Geometry check sheet. Reference: the model listing, model coordinates, mm. A direction names the side the tool comes from. Round coordinates to 2 decimals unless told otherwise and drop trailing zeros. Loops run counter-clockwise (first coordinate to the right, second up) from the corner with the lowest first, then second, coordinate; pieces in that order, holes last. Notation, with made-up numbers: (-33, -22.5) - (13, -22.5) arc R33 ccw to (13, 14.5) - close; hole circle Ø4 at (81.5, -21). An arc over 180 degrees is marked (long way). Answer in a Markdown table with one row per item. Add a question column.
Autodesk Inventor part; units mm, degrees
ref_plane "Work Plane2" through (3.35, 0, 0) normal (0, 0, -1) x (1, 0, 0)
ref_plane "YZ Plane" through (0, 0, 0) normal (1, 0, 0) x (0, 1, 0)
ref_plane "XZ Plane" through (0, 0, 0) normal (0, 1, 0) x (-1, 0, 0)
sketch "Szkic1" plane through (0, 0, 0) normal (0, 0, 1) x (1, 0, 0)
  line L0 (1.76, 0) -> (8, 0)
  line L1 (8, 0) -> (8, 1.5)
  line L2 (8, 1.5) -> (2.65, 1.5)
  line L3 (2.65, 1.5) -> (2.3433, 1.3466)
  line L4 (2.3433, 1.3466) -> (1.65, 1.3466)
  line L5 (0, 2.65) -> (0, 1.525)
  line L6 (0, 1.525) -> (1.2915, 0.8811)
  line L7 (1.2915, 0.8811) -> (1.76, 0)
  line L8 (-1.6, 0) -> (9.6, 0)
  line L9 (0, -0.53) -> (0, 3.18)
  line L10 (0, 2.65) -> (0.3466, 2.65)
  line L11 (0.3466, 2.65) -> (1.65, 1.3466)
  line L12 (2.65, 1.5) -> (1.4966, 1.5) construction
  dimension "d1" = 5.35
  dimension "d2" = 3
  dimension "d3" = 2.6933
  dimension "d4" = 3.05
  dimension "d5" = 26.5
  dimension "d6" = 62
  dimension "d7" = 1.76
  dimension "d8" = 0.3067
  dimension "d12" = 5.3
  dimension "d13" = 45
  dimension "d15" = 8
  dimension "d24" = 1.65
revolve "Bryła" add sketch "Szkic1" angle 360 about axis through (1.76, 0, 0) along (1, 0, 0) contours L7 L6 L5 L10 L11 L4 L3 L2 L1 L0
sketch "Szkic2" plane through (0, 0, 0) normal (-1, 0, 0) x (0, 0, 1)
  line L0 (0, 1.525) -> (0, 0) construction
  line L1 (0, 0) -> (1.525, 0) construction
  arc A0 (0.4575, 0) -> (0, 0.4575) centre (0, 0) ccw construction
  arc A1 (0.5338, 0) -> (0, 0.5337) centre (0, 0) ccw construction
  arc A2 (1.4843, 0.35) -> (0.35, 1.4843) centre (0, 0) ccw
  line L2 (0, 0) -> (1.0783, 1.0783) construction
  line L3 (0.35, 1.4843) -> (0.2734, 0.4584)
  line L4 (1.4843, 0.35) -> (0.4584, 0.2734)
  arc A3 (0.35, 1.4843) -> (0, 1.525) centre (0, 0) ccw
  arc A4 (1.525, 0) -> (1.4843, 0.35) centre (0, 0) ccw
  line L5 (0, -3.71) -> (0, 3.71)
  line L6 (-3.71, 0) -> (3.71, 0)
  arc A5 (0.35, -1.4843) -> (1.4843, -0.35) centre (0, 0) ccw
  line L7 (0.35, -1.4843) -> (0.2734, -0.4584)
  line L8 (1.4843, -0.35) -> (0.4584, -0.2734)
  arc A6 (0, -1.525) -> (0.35, -1.4843) centre (0, 0) ccw
  arc A7 (1.4843, -0.35) -> (1.525, 0) centre (0, 0) ccw
  arc A8 (-0.35, 1.4843) -> (-1.4843, 0.35) centre (0, 0) ccw
  line L9 (-0.35, 1.4843) -> (-0.2734, 0.4584)
  line L10 (-1.4843, 0.35) -> (-0.4584, 0.2734)
  arc A9 (0, 1.525) -> (-0.35, 1.4843) centre (0, 0) ccw
  arc A10 (-1.4843, 0.35) -> (-1.525, 0) centre (0, 0) ccw
  arc A11 (-0.35, -1.4843) -> (0, -1.525) centre (0, 0) ccw
  arc A12 (-1.4843, -0.35) -> (-0.35, -1.4843) centre (0, 0) ccw
  arc A13 (-1.525, 0) -> (-1.4843, -0.35) centre (0, 0) ccw
  line L11 (-1.4843, -0.35) -> (-0.4584, -0.2734)
  line L12 (-0.35, -1.4843) -> (-0.2734, -0.4584)
  arc A14 (0.2734, 0.4584) -> (0.4584, 0.2734) centre (0.4455, 0.4455) ccw
  arc A15 (0.4584, -0.2734) -> (0.2734, -0.4584) centre (0.4455, -0.4455) ccw
  arc A16 (-0.4584, 0.2734) -> (-0.2734, 0.4584) centre (-0.4455, 0.4455) ccw
  arc A17 (-0.2734, -0.4584) -> (-0.4584, -0.2734) centre (-0.4455, -0.4455) ccw
  point P0 (1.0783, -1.0783)
  point P1 (-1.0783, 1.0783)
  point P2 (-1.0783, -1.0783)
  dimension "d17" = 0.915
  dimension "d18" = 1.0675
  dimension "d19" = 3.05
  dimension "d20" = 45
  dimension "d21" = 0.35
extrude "Szczelina" add sketch "Szkic2" against normal up to next draft 5 contours L4 A14 L3 A2 | A5 L7 A15 L8 | L9 A16 L10 A8 | A12 L11 A17 L12
fillet "Zaokrąglenie1" radius 0.14 4 edges at (0, 1.525, 0) (0, 0, -1.525) (0, -1.525, 0) (0, 0, 1.525)
thread "Gwint"
chamfer "Faza1" distance 0.3067 distance2 0.1534 1 edges at (8, -1.5, 0) measured on face at (8, 0.3888, 0.4512)
ref_plane "Work Plane2" through (3.35, 0, 0) normal (0, 0, -1) x (1, 0, 0)
equation "\"d1\" = GEL"
equation "\"d2\" = GD"
equation "\"d3\" = BDM"
equation "\"d4\" = SDM"
equation "\"d7\" = INTI"
equation "\"d8\" = GAL"
equation "\"d12\" = KOD"
equation "\"d13\" = 0.5 * SEWI"
equation "\"d15\" = NLG"
equation "\"d24\" = KOH"
equation "\"d17\" = 0.3 * SDM"
equation "\"d18\" = 0.35 * SDM"
equation "\"d19\" = SDM"
equation "\"d21\" = 0.5 * SBR"
equation "\"d23\" = 0.2 * SBR"
equation "\"d10\" = GEL"
equation "\"d25\" = -0.5 * SPD + 0.5 * GD"
equation "\"d26\" = 0.5 * GAL"
equation "\"NLG\" = 8"
equation "\"GEL\" = 5.35"
equation "\"GAL\" = 0.61345 * PTC"
equation "\"SPD\" = NND - 1.2269 * PTC"
equation "\"KOD\" = 5.3"
equation "\"KOH\" = 1.65"
equation "\"SBR\" = 0.7"
equation "\"INTI\" = 1.76"
equation "\"SDM\" = 3.05"
equation "\"GD\" = NND"
equation "\"BDM\" = NND - GAL"
equation "\"SEWI\" = 90deg"
equation "\"d9\" = SDM"
equation "\"GUL\" = 0.61345 * PTC"
equation "\"TOA\" = 30deg"
equation "\"EPV\" = 3.15"
equation "\"THREADDIA\" = 3"
equation "\"RR\" = 0.3"
equation "\"PTC\" = 0.5"
equation "\"NND\" = 3"
equation "\"GD1\" = THREADDIA - 1.2269 * PTC"
properties part number "AS 1427 - M3 x 8" material "Stal, miękka"
Q1. Set-up check for faces 4 (the cylindrical face through (5.21, -1.5, -0.07)), 5 (the flat face through (0.573, -0.247, -0.779)), 6 (the flat face through (8, 0, 0)): record each of +Z, -Z, +X, -X, +Y, -Y from which the full face is reachable in a straight line by a thin tool's end or side.
Q2. Scan lines: line 1 (X direction, y = -1.6, z = -0.4); line 2 (Y direction, x = 3.5, z = 0.2); line 3 (Z direction, x = 1.5, y = 0.25). Record each from-to range of solid material in increasing order. Write a range as from..to.
Q3. Cross-section at A-A, the plane x = 1. Enter the section's corners in (y, z), plus the area to 3 significant figures.
Q4. Release check for a two-part mould opening along Y. For faces 1 (the flat face through (0.573, 0.779, 0.247)), 2 (the cylindrical face through (1.992, -1.345, -0.059)), 3 (the flat face through (0, 1, -1)) record: +Y half, -Y half, draft (parallel to the pull), parting line (faces both ways), or undercut.
Q5. Cross-section at B-B, the plane x = 3.75. Enter the section's corners in (y, z).
Q6. Depth check by flat-ended pin: P1, Ø1.5, axis at x = 4.5, z = -2, coming from the +Y side; P2, Ø1.5, axis at y = 1, z = -1.5, coming from the -X side; P3, Ø1, axis at x = 5, z = -0.5, coming from the -Y side. Enter the tip coordinate at first touch or a pass-through.
Check sheet entries:
| question | item | result |
|---|---|---|
| 1 | face 4 | +X |
| 1 | face 5 | -X |
| 1 | face 6 | +Z, -Z, +X, +Y, -Y |
| 2 | line 1 | 0..1.35 |
| 2 | line 2 | -1.49..1.49 |
| 2 | line 3 | -1.48..-0.21, 0.21..1.48 |
| 3 | outline | circle Ø3.99 at (0, 0); hole (-1, -0.23) - (-0.46, -0.19) arc R0.26 cw to (-0.19, -0.46) - (-0.23, -1) arc R1.03 ccw to (0.23, -1) - (0.19, -0.46) arc R0.26 cw to (0.46, -0.19) - (1, -0.23) arc R1.03 ccw to (1, 0.23) - (0.46, 0.19) arc R0.26 cw to (0.19, 0.46) - (0.23, 1) arc R1.03 ccw to (-0.23, 1) - (-0.19, 0.46) arc R0.26 cw to (-0.46, 0.19) - (-1, 0.23) arc R1.03 ccw to start |
| 3 | area | 11.0 mm² |
| 4 | face 1 | undercut |
| 4 | face 2 | parting line |
| 4 | face 3 | draft |
| 5 | outline | circle Ø3 at (0, 0) |
| 6 | P1 | y = 0.83 |
| 6 | P2 | x = 0 |
| 6 | P3 | y = -1.5 |
